Input: part model. Units: mm. Frame: model coordinates. Round coordinates to 2 decimals unless told otherwise and drop trailing zeros. Write each loop counter-clockwise with the first axis right and the second up, starting at its lowest first coordinate (ties: lowest second). Pieces come first, ordered by that corner, then holes. Notation, with made-up numbers: (74, 18.5) -> (78, 18.5) arc R26 cw to (78, 47.5) -> close; hole circle Ø11 at (-20, 17.25). An arc over 180 degrees is marked (long way). Write item = value, one per line. Start each with the question number.
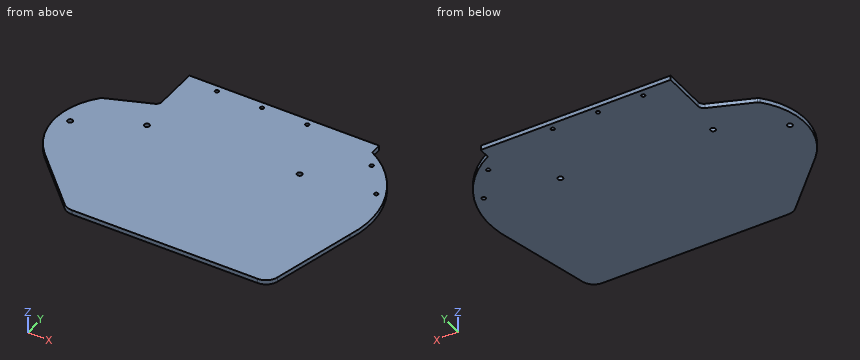
```python
from build123d import *

# Parameters (mm, degrees)
F1_DEPTH = 6.35
F2_R     = 2.579688
F3_DEPTH = 6.35
F4_R     = 3.571875
F5_DEPTH = 9.525
F6_R     = 2.667
F7_DEPTH = 7.62


with BuildPart() as f1:
    # F0 (on Top) → F1 (new body)
    with BuildSketch(Plane.XY):
        with BuildLine():
            Line((356.607027, 293.18534), (89.907027, 293.18534))
            Line((89.907027, 293.18534), (89.907027, 230.838141))
            ThreePointArc((89.907027, 230.838141), (88.528545, 226.367885), (84.871893, 223.450301))
            Line((84.871893, 223.450301), (25.612706, 200.169907))
            ThreePointArc((25.612706, 200.169907), (24.332233, 199.488924), (23.239671, 198.535164))
            ThreePointArc((23.239671, 198.535164), (-1.297086, 134.001926), (24.781553, 70.076219))
            Line((24.781553, 70.076219), (99.27516, -4.417388))
            ThreePointArc((99.27516, -4.417388), (105.455425, -8.546909), (112.745544, -9.997004))
            Line((112.745544, -9.997004), (373.810915, -9.997004))
            ThreePointArc((373.810915, -9.997004), (385.618685, -5.89622), (392.342874, 4.640625))
            Line((392.342874, 4.640625), (420.607724, 123.352996))
            ThreePointArc((420.607724, 123.352996), (416.146731, 211.779891), (356.607027, 277.31034))
            Line((356.607027, 277.31034), (356.607027, 293.18534))
        make_face()
    extrude(amount=F1_DEPTH)

    # F2 (on face) → F3 (cut, through all)
    with BuildSketch(Plane.XY.offset(6.35)):
        with Locations((261.357027, 283.66034)):
            Circle(F2_R)
        with Locations((197.857027, 283.66034)):
            Circle(F2_R)
        with Locations((134.357027, 283.66034)):
            Circle(F2_R)
    extrude(amount=-F3_DEPTH, mode=Mode.SUBTRACT)

    # F4 (on face) → F5 (cut)
    with BuildSketch(Plane.XY.offset(6.35)):
        with Locations((99.432027, 181.663465)):
            Circle(F4_R)
        with Locations((16.882027, 140.78534)):
            Circle(F4_R)
        with Locations((305.807027, 194.76034)):
            Circle(F4_R)
    extrude(amount=-F5_DEPTH, mode=Mode.SUBTRACT)

    # F6 (on face) → F7 (cut)
    with BuildSketch(Plane.XY.offset(6.35)):
        with Locations((370.04372, 254.438187)):
            Circle(F6_R)
        with Locations((404.631483, 208.943032)):
            Circle(F6_R)
    extrude(amount=-F7_DEPTH, mode=Mode.SUBTRACT)


solid = f1.part
```
1. Section B-B (y = 244). Output: boundary loops of the cut face in (x, z).
2. Pin query (flat end, axial travel): P1, Ø2, axis at x = 89, z = 1.5, coming from the -Y side; P2, Ø2, axis at x = 201.5, y = 46, coming from the -Z side; P3, Ø3, axis at y = 288, z = 2.5, coming from the +X side; P4, Ø1, axis at y = 147, z = 3, coming from the +X side. Return the tip coordinate at first contact, or that it passes through.
3. Section A-A (z = 2.25). State how many separate pieces and enclosed holes the cut face has, then the cut area to 3 significant figures.
4. Line query: line 1 along Y through (x, z) = (99.5, 5); line 2 along Y through (x, z) = (91.5, 5.5); line 3 along X through (y, z) = (140, 5.75). Output: solid intervals per line, ascending.
5. Section C-C (x = 35). Output: boundary loops of the cut face in (y, z), then the cut area to 3 significant figures.
Check sheet entries:
q1.outline = (89.91, 0) -> (396.96, 0) -> (396.96, 6.35) -> (89.91, 6.35) -> close
q2.P1 = 4.86
q2.P2 = 0
q2.P3 = 356.61
q2.P4 = 425.48
q3.separate_pieces = 1
q3.enclosed_holes = 8
q3.area = 109,000 mm2
q4.line_1 = -4.64 to 178.09, 185.23 to 293.19
q4.line_2 = 3.36 to 293.19
q4.line_3 = -1.18 to 13.4, 20.37 to 424.47
q5.outline = (59.86, 0) -> (203.86, 0) -> (203.86, 6.35) -> (59.86, 6.35) -> close
q5.area = 914 mm2
